from build123d import *

# Parameters (mm, degrees)
BASE_FLANGE1_DEPTH              = 30
F_3_0MM_PRESS_DOWEL_HOLE1_D     = 3
F_3_0MM_PRESS_DOWEL_HOLE2_D     = 3
F_3_0MM_PRESS_DOWEL_HOLE3_D     = 3
F_3_0MM_PRESS_DOWEL_HOLE3_DEPTH = 6
F_3_0MM_PRESS_DOWEL_HOLE3_TIP   = 0.901290929


# Sheet-metal steps are written as plain solids
with BuildPart() as part:
    # Sketch2 → Base-Flange1 (new body)
    with BuildSketch(Plane(origin=(0, 0, 0), x_dir=(1, 0, 0), z_dir=(0, 1, 0))):
        with BuildLine():
            Line((0, 0), (0, 72.7634))
            ThreePointArc((0, 72.7634), (0.655084973, 74.344915027), (2.2366, 75))
            Line((2.2366, 75), (10, 75))
            Line((10, 75), (10, 73.5))
            Line((10, 73.5), (2.2366, 73.5))
            ThreePointArc((2.2366, 73.5), (1.715745145, 73.284254855), (1.5, 72.7634))
            Line((1.5, 72.7634), (1.5, 0))
            Line((1.5, 0), (0, 0))
        make_face()
    extrude(amount=BASE_FLANGE1_DEPTH)

    # Ø3.0mm Press Dowel Hole1 (through all)
    with Locations(Plane(origin=(0, 0, -75), x_dir=(-1, 0, 0), z_dir=(0, 0, -1))):
        with Locations((-6.667186687, 15)):
            Hole(F_3_0MM_PRESS_DOWEL_HOLE1_D / 2)

    # Ø3.0mm Press Dowel Hole2 (through all)
    with Locations(Plane.ZY):
        with Locations((-10, 15)):
            Hole(F_3_0MM_PRESS_DOWEL_HOLE2_D / 2)

    # Ø3.0mm Press Dowel Hole3
    with Locations(Plane(origin=(-82.525513363, 241.531359221, -81), x_dir=(1, 0, 0), z_dir=(0, 0, -1))):
        with Locations((220.525513363, 156.531359221), (102.525513363, 181.531359221), (102.525513363, 271.531359221), (89.19270005, 226.531359221), (210.525513363, 317.793651488), (230.525513363, 317.793651488), (252.525513363, 320.462332131), (232.525513363, 300.462332131), (252.525513363, 132.600386311), (232.525513363, 152.600386311), (111.286271896, 136.531359221), (91.286271896, 136.531359221), (41.525513363, 196.432813402), (13.525513363, 196.432813402), (41.525513363, 138.767959221), (13.525513363, 138.767959221), (41.525513363, 256.62990504), (13.525513363, 256.62990504), (41.525513363, 314.294759221), (13.525513363, 314.294759221)):
            Hole(F_3_0MM_PRESS_DOWEL_HOLE3_D / 2, depth=F_3_0MM_PRESS_DOWEL_HOLE3_DEPTH)
            with Locations((0, 0, -(F_3_0MM_PRESS_DOWEL_HOLE3_DEPTH + F_3_0MM_PRESS_DOWEL_HOLE3_TIP / 2))):  # 118° drill point
                Cone(0, F_3_0MM_PRESS_DOWEL_HOLE3_D / 2, F_3_0MM_PRESS_DOWEL_HOLE3_TIP, mode=Mode.SUBTRACT)


solid = part.part
Geometry: final body of the model. Coordinates: model frame, mm. A direction names the side the tool comes from. Give positions to 0.01 mm unless a question says otherwise; leave off trailing zeros. Write each loop counter-clockwise with the first axis right and the second up, starting at its lowest first coordinate (ties: lowest second). Pieces come first, ordered by that corner, then holes.
(1) First-contact query: P1, Ø4, axis at y = 15, z = -10, coming from the +X side. Flat tip, straight axial feed; report the tip coordinate or a pass-through.
(2) Cut plane C-C, the plane x = 7.25. Return loops of the section in (y, z).
(3) Access query for faces 5 (the flat face through (1.5, 15, -37)), 6 (the flat face through (0, 15, -36)). Directions: +Z, -Z, +X, -X, +Y, -Y. A direction counts if a zero-diameter tool reaches every point of the face in a straight line with its end or side. Return the directions, or none.
(4) Cut plane B-B, the plane z = -10. Return loops of the section in (x, y).
(5) Mould query, pull axis Y, two halves, no side actions, for faces 1 (the cylindrical face through (8.1, 15.45, -74.24)), 2 (the flat face through (1, 0, -43)), 3 (the cylindrical face through (0.76, 15.07, -8.5)), 4 (the flat face through (1, 15, 0)). Classes: released by +Y, released by -Y, zero draft, split by the parting line, or undercut.
(6) Ray query, line 1 (Y direction, x = 0.7, z = -10); line 2 (X direction, y = 19, z = -25); line 3 (Z direction, x = 8.5, y = 14.75). Return the intervals inside material, ascending.
(7) Cut plane A-A, the plane y = 15. Return loops of the section in (x, z), then the cut area to 3 significant figures.
(8) Cut plane D-D, the plane y = 22.75. Return loops of the section in (x, z).
Values follow:
1. P1: stops at x = 1.5
2. outline: (0, -75) - (13.62, -75) - (13.62, -73.5) - (0, -73.5) - close; (16.38, -75) - (30, -75) - (30, -73.5) - (16.38, -73.5) - close
3. face 5: +Z, +X, +Y, -Y
3. face 6: +Z, -Z, -X, +Y, -Y
4. outline: (0, 0) - (1.5, 0) - (1.5, 13.5) - (0, 13.5) - close; (0, 16.5) - (1.5, 16.5) - (1.5, 30) - (0, 30) - close
5. face 1: undercut
5. face 2: released by -Y
5. face 3: undercut
5. face 4: zero draft
6. line 1: y = 0 to 13.5, 16.5 to 30
6. line 2: x = 0 to 1.5
6. line 3: z = -75 to -73.5
7. outline: (0, -72.76) arc R2.24 ccw to (2.24, -75) - (5.17, -75) - (5.17, -73.5) - (2.24, -73.5) arc R0.74 cw to (1.5, -72.76) - (1.5, -11.5) - (0, -11.5) - close; (0, -8.5) - (1.5, -8.5) - (1.5, 0) - (0, 0) - close; (8.17, -75) - (10, -75) - (10, -73.5) - (8.17, -73.5) - close
7. area: 115 mm2
8. outline: (0, -72.76) arc R2.24 ccw to (2.24, -75) - (10, -75) - (10, -73.5) - (2.24, -73.5) arc R0.74 cw to (1.5, -72.76) - (1.5, 0) - (0, 0) - close
